Build history of the part. All positions in model axes, mm. Face numbers are marked on the shaded views. Give positions to 0.01 mm unless a question says otherwise; leave off trailing zeros. Loops run counter-clockwise (first coordinate to the right, second up) from the corner with the lowest first, then second, coordinate; pieces in that order, holes last. Notation, with made-up numbers: M -20.5,-24 L -13.5,-24 A11 cw -13.5,-19 Z; hole C 60,36.5 d11. An arc over 180 degrees is marked long. Answer as a JSON object with one key per item and string values. Group by question number.
1. Mould opens along Z. For the marked faces 1, 2 and 3 say: released by +Z, released by -Z, zero draft, split by the parting line, or undercut.
2. Drill centre lines: line 1 along X through (y, z) = (-0.5, -0.75); line 2 along Y through (x, z) = (25, 0); line 3 along X through (y, z) = (-2, -1.75). Where is each one in solid material? Low to high. Write a range as [from, to].
3. Slice it at A-A (x = 17.5). List the corners of the cut face in (y, z).
4. Drop flat-ended pins along their axis: pin 1 Ø1.6 at (x, z) = (0.5, 0) entering from -Y; pin 2 Ø0.7 at (x, z) = (0.5, -0.5) entering from +Y; pin 3 Ø1.5 at (x, z) = (17.5, 2.5) entering from +Y. Give the stop position or say it passes through.
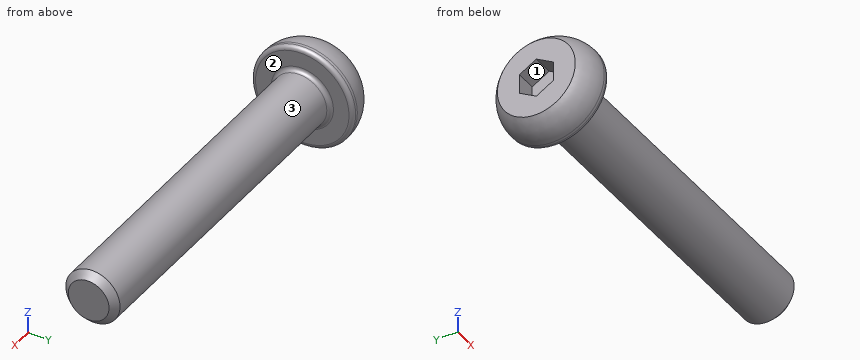
from build123d import *

# Parameters (mm, degrees)
CUT_EXTRUDE_1_DEPTH = 1.5
FILLET_1_R          = 0.3
CHAMFER_1_SIZE      = 0.5


with BuildPart() as part:
    # Эскиз1 → Повернуть1 (revolve)
    with BuildSketch(Plane.XY):
        with BuildLine():
            Line((0, 0), (0, 2.875))
            ThreePointArc((0, 2.875), (0.908484425, 3.521678457), (2, 3.75))
            Line((2, 3.75), (2.5, 3.75))
            Line((2.5, 3.75), (2.5, 2))
            Line((2.5, 2), (27.5, 2))
            Line((27.5, 2), (27.5, 0))
            Line((27.5, 0), (0, 0))
        make_face()
    revolve(axis=Axis((27.5, 0, 0), (-1, 0, 0)))

    # Эскиз2 → Вырез-Вытянуть1 (cut)
    with BuildSketch(Plane.ZY):
        Polygon((0.721687836, 1.25), (-0.721687836, 1.25), (-1.443375673, 0), (-0.721687836, -1.25), (0.721687836, -1.25), (1.443375673, 0), align=None)
    extrude(amount=-CUT_EXTRUDE_1_DEPTH, mode=Mode.SUBTRACT)

    # Скругление1
    fillet_1_edges = [part.edges().sort_by_distance(p)[0] for p in [
        (2.5, -2, 0),
        (2.5, -3.75, 0),
    ]]
    fillet(fillet_1_edges, radius=FILLET_1_R)

    # Фаска1
    chamfer_1_edges = [part.edges().sort_by_distance(p)[0] for p in [
        (27.5, -2, 0),
    ]]
    chamfer(chamfer_1_edges, length=CHAMFER_1_SIZE)


solid = part.part
Established:
{
 "1": {"face 1": "undercut", "face 2": "zero draft", "face 3": "split by the parting line"},
 "2": {"line 1": "x = [1.5, 27.5]", "line 2": "y = [-2, 2]", "line 3": "x = [0, 2.5]"},
 "3": {"outline": "C 0,0 d4"},
 "4": {"pin 1": "stops at y = -3.66", "pin 2": "stops at y = 3.47", "pin 3": "stops at y = 0.97"}
}
